Design review of the part built by this model. Coordinates are the model's own, in mm. Face numbers are marked on the shaded views. A direction names the side the tool comes from. Coordinates: 2 decimals unless noted, no trailing zeros. Write each loop counter-clockwise with the first axis right and the second up, starting at its lowest first coordinate (ties: lowest second). Pieces come first, ordered by that corner, then holes.
Q1. Clearance check with flat-ended pins moving along their axes: pin 1 Ø3 at (x, y) = (10.5, -117.5) entering from -Z; pin 2 Ø21 at (x, y) = (47, -294.5) entering from -Z; pin 3 Ø4 at (x, z) = (42, -79) entering from -Y. State where each tip first meets the part, or that it passes through.
Q2. The part is to be moulded in two halves that separate along Z. For the marked faces 4, 5 and 6, say which applies: +Z half, -Z half, draft (parallel to the pull), parting line (faces both ways), or undercut.
Q3. Machinability: for the marked faces 1, 2 and 3, which of the approach directions +Z, -Z, +X, -X, +Y, -Y give a long, thin tool a straight path to every point of the face, cutting with its end or side? Answer none if there is none.
Q4. Add section D-D, the plane y = -547. Give the boundary of the cut face in (x, z).
Q5. To check wall thickness, follow probe 1 along Z at (x, y) = (55.5, -65); probe 2 along Y at (x, z) = (22, -18); probe 3 along Y at (x, z) = (23.5, -34.5). State the ranges of each line that lie inside material, in increasing order.
Q6. Add section B-B, the plane z = -45. Give the boundary of the cut face in (x, y).
Q7. Add section A-A, the plane x = 35. Give the boundary of the cut face in (y, z), plus the area to 3 significant figures.
Q8. Add section C-C, the plane y = -380.5. Give the boundary of the cut face in (x, z), plus the area to 3 significant figures.
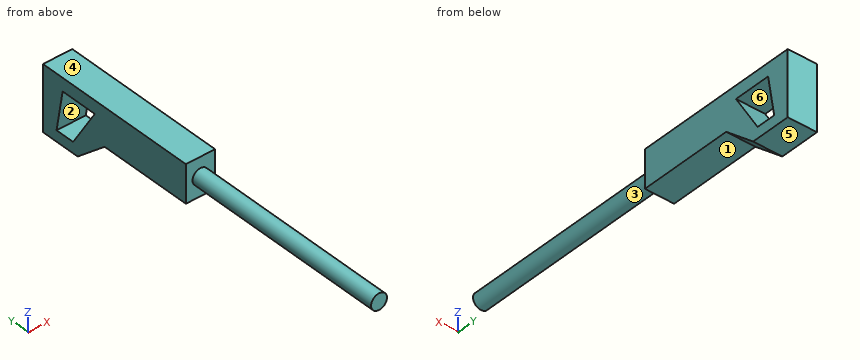
from build123d import *

# Parameters (mm, degrees)
BOSS_EXTRUDE1_DEPTH     = 70
CUT_EXTRUDE1_DEPTH      = 435.655035632
CUT_EXTRUDE1_DEPTH_BACK = 435.655035632
SKETCH4_R               = 19.05
BOSS_EXTRUDE2_DEPTH     = 500


with BuildPart() as part:
    # Sketch2 → Boss-Extrude1 (new body)
    with BuildSketch(Plane(origin=(0, 0, 0), x_dir=(0, 0, -1), z_dir=(1, 0, 0))):
        Polygon((0, 0), (155, 0), (155, -97.047904462), (90, -172.424894861), (90, -400), (0, -400), align=None)
    extrude(amount=BOSS_EXTRUDE1_DEPTH)

    # Sketch3 → Cut-Extrude1 (cut, two sides: drawn at the far end of the back side and taken through both)
    with BuildSketch(Plane(origin=(70, 0, 0), x_dir=(0, 0, -1), z_dir=(1, 0, 0)).offset(-CUT_EXTRUDE1_DEPTH_BACK)):
        Polygon((31, -55), (129, -38), (129, -84.32322248), (31, -145), align=None)
    extrude(amount=CUT_EXTRUDE1_DEPTH + CUT_EXTRUDE1_DEPTH_BACK, mode=Mode.SUBTRACT)

    # Sketch4 → Boss-Extrude2 (add)
    with BuildSketch(Plane.XZ.offset(400)):
        with Locations(Location((35, -45, 0), (0, 0, 270))):
            Circle(SKETCH4_R)
    extrude(amount=BOSS_EXTRUDE2_DEPTH)


solid = part.part
Here are the results:
1. pin 1: stops at z = -138.66
1. pin 2: stops at z = -90
1. pin 3: stops at y = -400
2. face 4: +Z half
2. face 5: -Z half
2. face 6: undercut
3. face 1: -Z, +X, -X, -Y
3. face 2: +X, -X
3. face 3: -Y
4. outline: circle Ø38.1 at (35, -45)
5. probe 1: z = -155 to -129, -31 to 0
5. probe 2: y = -400 to 0
5. probe 3: y = -900 to -142.83, -54.39 to 0
6. outline: (0, -400) - (15.95, -400) - (15.95, -900) - (54.05, -900) - (54.05, -400) - (70, -400) - (70, -136.33) - (0, -136.33) - close; (0, -52.57) - (70, -52.57) - (70, 0) - (0, 0) - close
7. outline: (-900, -64.05) - (-400, -64.05) - (-400, -90) - (-172.42, -90) - (-97.05, -155) - (0, -155) - (0, 0) - (-400, 0) - (-400, -25.95) - (-900, -25.95) - close; hole (-145, -31) - (-84.32, -129) - (-38, -129) - (-55, -31) - close
7. area: 57,100 mm2
8. outline: (0, -90) - (70, -90) - (70, 0) - (0, 0) - close
8. area: 6,300 mm2
